The listing builds one solid part. Answer for the finished solid, in the listing's coordinates (mm). A direction names the side the tool comes from. Give positions to 0.01 mm unless a question says otherwise; leave off trailing zeros. Write each loop counter-clockwise with the first axis right and the second up, starting at its lowest first coordinate (ties: lowest second). Pieces come first, ordered by that corner, then holes. Notation, with made-up numbers: (2.25, 7.25) - (22.25, 7.25) arc R19 ccw to (22.25, 23.25) - close; hole circle Ø3 at (-18, 86.25). An arc over 180 degrees is marked (long way). One line per item, written item: value. Start each with the question number.
from build123d import *

# Parameters (mm, degrees)
F0_W     = 10
F0_H     = 3
F2_W     = 400
F2_H     = 400
F2_R     = 10
F3_DEPTH = 3
F6_R     = 9
F7_DEPTH = 120
F8_R     = 150
F9_DEPTH = 200


with BuildPart() as f1:
    # F0 (on Front) → F1 (revolve)
    with BuildSketch(Plane.XZ):
        Polygon((-175, 5), (-150, 5), (-150, 55), (-151, 55), (-151, 95), (-174, 95), (-174, 55), (-175, 55), align=None)
        Polygon((-10, 5), (-150, 5), (-175, 5), (-175, 2), (-10, 2), align=None)
        with Locations((-5, 3.5)):
            Rectangle(F0_W, F0_H)
    revolve(axis=Axis((0, 0, 187.9212413023), (0, 0, -1)))

    # F2 (on Top) → F3 (join)
    with BuildSketch(Plane.XY):
        Rectangle(F2_W, F2_H)
        with Locations((-170, -170)):
            Circle(F2_R, mode=Mode.SUBTRACT)
        with Locations((170, -170)):
            Circle(F2_R, mode=Mode.SUBTRACT)
        with Locations((-170, 170)):
            Circle(F2_R, mode=Mode.SUBTRACT)
        with Locations((170, 170)):
            Circle(F2_R, mode=Mode.SUBTRACT)
    extrude(amount=F3_DEPTH)

    # F4 (on Front) → F5 (revolve)
    with BuildSketch(Plane.XZ):
        Polygon((249.6194698092, 41.5098406888), (150, 50.2254149636), (149.9128442573, 49.2292202655), (249.5323140664, 40.5136459907), align=None)
    revolve(axis=Axis((262.7442754949, 0, 30.3233706049), (0.9961946981, 0, -0.0871557427)))

    # F6 (on face) → F7 (cut)
    with BuildSketch(Plane(origin=(244.1192753946, 0, -21.3576691452), x_dir=(0, 1, 0), z_dir=(0.9961946981, 0, -0.0871557427))):
        with Locations((0, 53.1076535083)):
            Circle(F6_R)
    extrude(amount=-F7_DEPTH, mode=Mode.SUBTRACT)

    # F8 (on face) → F9 (cut)
    with BuildSketch(Plane.XY.offset(5)):
        Circle(F8_R)
    extrude(amount=F9_DEPTH, mode=Mode.SUBTRACT)


solid = f1.part
Item 1: Straight lines are drawn through the part: line 1 along Y through (x, z) = (-170, 1.05); line 2 along Y through (x, z) = (0, 80.5); line 3 along Z through (x, y) = (-142, 13.5). For each, find the intervals that lie inside material, in ascending order.
Item 2: Find section A-A on y = 0. Determine the outline of the cut face in (x, z), plus the area to 3 significant figures.
Item 3: For faces 4 (the cylindrical face through (-144.027, 45.356, 75.28)), 5 (the cylindrical face through (179.237, -173.83, 1.479)), determine the directions among +Z, -Z, +X, -X, +Y, -Y from which every point of the face is accessible in a straight line to the end or side of a thin tool.
Item 4: The mould has two halves that part along Y. Classify faces 1 (the cylindrical face through (-138.562, 57.451, 29.65)), 2 (the cylindrical face through (22.65, 172.52, 74.72)), 3 (the flat face through (-52, 143, 95)): +Y half, -Y half, draft (parallel to the pull), parting line (faces both ways), or undercut.
Item 5: Each of these flat-tipped pins is pushed along its axis until it touches: pin 1 Ø16 at (x, y) = (170, 170) entering from +Z; pin 2 Ø2 at (y, z) = (67.5, 53) entering from +X; pin 3 Ø4 at (y, z) = (-69.5, 72) entering from +X; pin 4 Ø8 at (x, z) = (159, 11) entering from +Y. Where does it stop, or does it pass through?
Item 6: Find section C-C on x = 128. Determine the outline of the cut face in (y, z).
Item 7: Find section D-D on y = 70.5. Determine the outline of the cut face in (x, z), plus the area to 3 significant figures.
Item 8: Find section B-B on z = 76.5. Determine the outline of the cut face in (x, y), plus the area to 3 significant figures.
Values:
1. line 1: -200 to -180, -160 to 160, 180 to 200
1. line 2: -174 to -151, 151 to 174
1. line 3: 0 to 5
2. outline: (-200, 0) - (200, 0) - (200, 3) - (175, 3) - (175, 27.96) - (247.88, 21.59) - (247.96, 22.58) - (150, 31.15) - (150, 5) - (-150, 5) - (-150, 55) - (-151, 55) - (-151, 95) - (-174, 95) - (-174, 55) - (-175, 55) - (-175, 3) - (-200, 3) - close; (150, 49.22) - (249.53, 40.51) - (249.62, 41.51) - (175, 48.04) - (175, 55) - (174, 55) - (174, 95) - (151, 95) - (151, 55) - (150, 55) - close
2. area: 5,940 mm^2
3. face 4: +Z
3. face 5: +Z, -Z
4. face 1: undercut
4. face 2: parting line
4. face 3: draft
5. pin 1: through
5. pin 2: x = 161.87
5. pin 3: x = 160.37
5. pin 4: y = 81.24
6. outline: (-200, 0) - (200, 0) - (200, 3) - (119.34, 3) - (119.34, 55) - (117.86, 55) - (117.86, 95) - (80.11, 95) - (80.11, 55) - (78.2, 55) - (78.2, 5) - (-78.2, 5) - (-78.2, 55) - (-80.11, 55) - (-80.11, 95) - (-117.86, 95) - (-117.86, 55) - (-119.34, 55) - (-119.34, 3) - (-200, 3) - close
7. outline: (-200, 0) - (200, 0) - (200, 3) - (160.17, 3) - (160.17, 55) - (159.08, 55) - (159.08, 95) - (133.53, 95) - (133.53, 55) - (132.4, 55) - (132.4, 5) - (-132.4, 5) - (-132.4, 55) - (-133.53, 55) - (-133.53, 95) - (-159.08, 95) - (-159.08, 55) - (-160.17, 55) - (-160.17, 3) - (-200, 3) - close
7. area: 6,660 mm^2
8. outline: circle Ø348 at (0, 0); hole circle Ø302 at (0, 0)
8. area: 23,500 mm^2
